```python
from build123d import *

# Parameters (mm, degrees)
F0_R        = 1.5
F0_R_2      = 1.6
F1_DEPTH    = 3
F2_SIZE     = 2
F3_R        = 4.1
F4_DEPTH    = 4
F5_T4_DEPTH = 40.5734639037
F6_T1_DEPTH = 9.1433659759
F6_T3_DEPTH = 10
F6_T6_ANGLE = 90
F6_T8_ANGLE = 90


# Not quite as in the source:
# - a fillet or chamfer that OpenCascade refuses, or shapes differently, is made with other operations: its cross-section is extruded or revolved along the edge and cut away or added


with BuildPart() as f1:
    # F0 (on Top) → F1 (new body)
    with BuildSketch(Plane.XY):
        with BuildLine():
            Line((22, 10), (-22, 10))
            ThreePointArc((-22, 10), (-25.5355339059, 8.5355339059), (-27, 5))
            Line((-27, 5), (-27, -5))
            ThreePointArc((-27, -5), (-25.5355339059, -8.5355339059), (-22, -10))
            Line((-22, -10), (22, -10))
            ThreePointArc((22, -10), (25.5355339059, -8.5355339059), (27, -5))
            Line((27, -5), (27, 5))
            ThreePointArc((27, 5), (25.5355339059, 8.5355339059), (22, 10))
        make_face()
        with Locations((-15, 0)):
            Circle(F0_R, mode=Mode.SUBTRACT)
        with Locations((4, 0)):
            Circle(F0_R, mode=Mode.SUBTRACT)
        with Locations((21, 0)):
            Circle(F0_R_2, mode=Mode.SUBTRACT)
    extrude(amount=F1_DEPTH)

    # F2
    f2_edges = [f1.edges().sort_by_distance(p)[0] for p in [
        (-16.5, 0, 3),
        (2.5, 0, 3),
    ]]
    chamfer(f2_edges, length=F2_SIZE)

    # F3 (on face) → F4 (join)
    with BuildSketch(Plane(origin=(0, 0, 0), x_dir=(1, 0, 0), z_dir=(0, 0, -1))):
        with BuildLine():
            Line((14, 10), (14, -10))
            Line((14, -10), (22, -10))
            ThreePointArc((22, -10), (25.5355339059, -8.5355339059), (27, -5))
            Line((27, -5), (27, 5))
            ThreePointArc((27, 5), (25.5355339059, 8.5355339059), (22, 10))
            Line((22, 10), (14, 10))
        make_face()
        with Locations((21, 0)):
            Circle(F3_R, mode=Mode.SUBTRACT)
    extrude(amount=F4_DEPTH)

    # F5: chamfer of 4 on 1 edges, made by hand


with BuildPart() as f5_tool2:
    # F5_s3 → F5_t4 (new body)
    with BuildSketch(Plane.XZ.offset(20.2867319519)):
        Polygon((18, -4), (14, 0), (14, -4), align=None)
    extrude(amount=-F5_T4_DEPTH)

    split(bisect_by=Plane.XY, keep=Keep.BOTTOM)


with BuildPart() as f1_1:
    add(f1.part)

    # F5_t1: cut F5_tool2
    add(f5_tool2.part, mode=Mode.SUBTRACT)

    # F6: chamfer of 2 on 5 edges, made by hand

    # F6_s2 → F6_t1 (cut)
    with BuildSketch(Plane.YZ.offset(12.8566340241)):
        Polygon((-10, -2), (-8, -4), (-10, -4), align=None)
        Polygon((10, -2), (8, -4), (10, -4), align=None)
    extrude(amount=F6_T1_DEPTH, mode=Mode.SUBTRACT)

    # F6_s4 → F6_t3 (cut)
    with BuildSketch(Plane.XZ.offset(-5)):
        Polygon((27, -2), (25, -4), (27, -4), align=None)
    extrude(amount=F6_T3_DEPTH, mode=Mode.SUBTRACT)

    # F6_s5 → F6_t6 (revolve, cut)
    with BuildSketch(Plane.XZ.offset(5)):
        Polygon((27, -2), (25, -4), (27, -4), align=None)
    revolve(axis=Axis((22, -5, -4), (0, 0, -1)), revolution_arc=F6_T6_ANGLE, mode=Mode.SUBTRACT)

    # F6_s7 → F6_t8 (revolve, cut)
    with BuildSketch(Plane.YZ.offset(22)):
        Polygon((10, -2), (8, -4), (10, -4), align=None)
    revolve(axis=Axis((22, 5, -4), (0, 0, -1)), revolution_arc=F6_T8_ANGLE, mode=Mode.SUBTRACT)


solid = f1_1.part
```
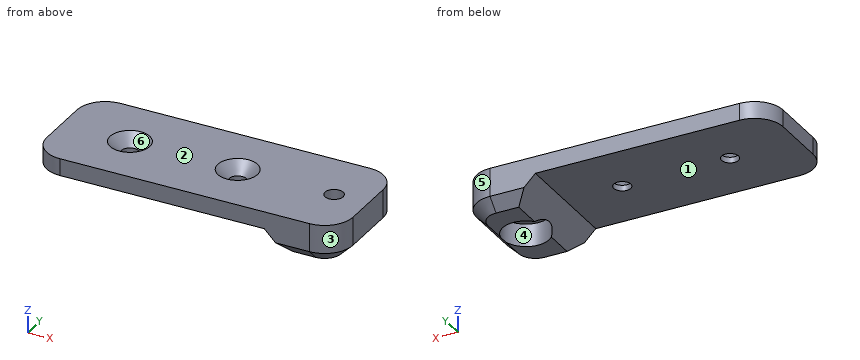
Check sheet for the modelled part. Datum: model origin and axes. Units: mm. Face numbers are marked on the shaded views. A direction names the side the tool comes from. Round coordinates to 2 decimals unless told otherwise and drop trailing zeros. Order: outer loops, then holes, each group sorted by start corner. A loop starts at its lowest first (then second) coordinate and runs counter-clockwise, first axis right, second up. Notation, with made-up numbers: (51.25, 87) - (108.25, 87) arc R33 ccw to (108.25, 122) - close; hole circle Ø2 at (30, 76). An arc over 180 degrees is marked (long way). Answer as CSV lines item,"result". Start each with the question number.
1) Draft check along Y on the marked faces 3, 4, 5 and 6. Enter one of: +Y half, -Y half, draft (parallel to the pull), parting line (faces both ways), or undercut.
2) Section check C-C (z = -1.25). Record the cut outline in (x, y), then the cut area to 3 significant figures.
3) Tool access check on the marked faces 1 and 2. Record the directions out of +Z, -Z, +X, -X, +Y, -Y that give a thin tool (end or side, any length) a straight path to the whole face; none if there is none.
4) Scan lines: probe 1 along Y at (x, z) = (-15, 0.45); probe 2 along X at (y, z) = (-0.5, 1.5); probe 3 along Z at (x, y) = (-4, -9). Record each from-to range of solid material in increasing order.
5) Section check A-A (y = 0). Record the cut outline in (x, z).
6) Section check B-B (x = 21). Record the cut outline in (y, z), then the cut area to 3 significant figures.
7) Depth check by flat-ended pin: pin 1 (1 mm diameter, centred on y = -4.5, z = -1, fed in from -X); pin 2 (9.5 mm diameter, centred on x = 21, y = 0, fed in from +Z); pin 3 (1.8 mm diameter, centred on x = -15, y = 0, fed in from -Z); pin 4 (2 mm diameter, centred on x = -8.5, y = -6.5, fed in from -Z). Enter the tip coordinate at first touch or a pass-through.
8) Section check D-D (x = 4). Record the cut outline in (y, z), then the cut area to 3 significant figures.
Determined:
1,face 3,"-Y half"
1,face 4,"undercut"
1,face 5,"+Y half"
1,face 6,"undercut"
2,outline,"(15.25, -10) - (22, -10) arc R5 ccw to (27, -5) - (27, 5) arc R5 ccw to (22, 10) - (15.25, 10) - close; hole circle Ø8.2 at (21, 0)"
2,area,"171 mm^2"
3,face 1,"-Z, -X, +Y, -Y"
3,face 2,"+Z, +X, -X, +Y, -Y"
4,probe 1,"-10 to -1.5, 1.5 to 10"
4,probe 2,"-27 to -16.94, -13.06 to 2.06, 5.94 to 19.48, 22.52 to 27"
4,probe 3,"0 to 3"
5,outline,"(-27, 0) - (-16.5, 0) - (-16.5, 1) - (-18.5, 3) - (-27, 3) - close; (-13.5, 0) - (2.5, 0) - (2.5, 1) - (0.5, 3) - (-11.5, 3) - (-13.5, 1) - close; (5.5, 0) - (14, 0) - (16.9, -2.9) - (16.9, 0) - (19.4, 0) - (19.4, 3) - (7.5, 3) - (5.5, 1) - close; (22.6, 0) - (25.1, 0) - (25.1, -3.9) - (27, -2) - (27, 3) - (22.6, 3) - close"
6,outline,"(-10, -2) - (-8, -4) - (-4.1, -4) - (-4.1, 0) - (-1.6, 0) - (-1.6, 3) - (-10, 3) - close; (1.6, 0) - (4.1, 0) - (4.1, -4) - (8, -4) - (10, -2) - (10, 3) - (1.6, 3) - close"
6,area,"93.6 mm^2"
7,pin 1,"x = 14.5"
7,pin 2,"z = 3"
7,pin 3,"through"
7,pin 4,"z = 0"
8,outline,"(-10, 0) - (-1.5, 0) - (-1.5, 1) - (-3.5, 3) - (-10, 3) - close; (1.5, 0) - (10, 0) - (10, 3) - (3.5, 3) - (1.5, 1) - close"
8,area,"47.0 mm^2"
